```python
from build123d import *

# Parameters (mm, degrees)
BOSS_EXTRUDE1_DEPTH = 28.3
SKETCH2_W           = 52.78
SKETCH2_H           = 15.38
CUT_EXTRUDE1_DEPTH  = 10.2
CUT_EXTRUDE2_START  = 28.3
SKETCH2_2_W         = 52.78
SKETCH2_2_H         = 15.38
CUT_EXTRUDE2_DEPTH  = 10.2
CUT_EXTRUDE3_REACH  = 69.103
SKETCH3_R           = 1.65
BOSS_EXTRUDE2_START = 11.1
BOSS_EXTRUDE2_DEPTH = 3.4
CUT_EXTRUDE4_DEPTH  = 4.02
SKETCH6_R           = 1.65
BOSS_EXTRUDE3_DEPTH = 3.2
CUT_EXTRUDE5_DEPTH  = 4.22
SKETCH10_W          = 41.62
SKETCH10_H          = 8.42
CUT_EXTRUDE6_DEPTH  = 1


with BuildPart() as part:
    # Sketch1 → Boss-Extrude1 (new body)
    with BuildSketch(Plane.XY):
        with BuildLine():
            Line((0, 21.81), (3.19, 21.81))
            Line((3.19, 21.81), (3.19, 4.02))
            Line((3.19, 4.02), (53.61, 4.02))
            Line((53.61, 4.02), (53.61, 21.81))
            Line((53.61, 21.81), (56.8, 21.81))
            Line((56.8, 21.81), (56.8, 2))
            ThreePointArc((56.8, 2), (56.214213562, 0.585786438), (54.8, 0))
            Line((54.8, 0), (2, 0))
            ThreePointArc((2, 0), (0.585786438, 0.585786438), (0, 2))
            Line((0, 2), (0, 21.81))
        make_face()
    extrude(amount=BOSS_EXTRUDE1_DEPTH)

    # Sketch2 → Cut-Extrude1 (cut)
    with BuildSketch(Plane.XY):
        with Locations((28.4, 11.71)):
            Rectangle(SKETCH2_W, SKETCH2_H)
    extrude(amount=CUT_EXTRUDE1_DEPTH, mode=Mode.SUBTRACT)

    # Sketch2<2> → Cut-Extrude2 (cut)
    with BuildSketch(Plane.XY.offset(CUT_EXTRUDE2_START)):
        with Locations((28.4, 11.71)):
            Rectangle(SKETCH2_2_W, SKETCH2_2_H)
    extrude(amount=-CUT_EXTRUDE2_DEPTH, mode=Mode.SUBTRACT)

    # Cut-Extrude3: up to this face of the body (flat: up to its plane)
    cut_extrude3_end = Plane(part.part.faces().sort_by_distance((56.8, 11.905, 14.15))[0])
    # Sketch3 → Cut-Extrude3 (cut, up to the picked face)
    with BuildSketch(Plane.ZY, mode=Mode.PRIVATE) as cut_extrude3_sk1:
        with Locations((3.9, 8.91)):
            Circle(SKETCH3_R)
    cut_extrude3_tool1 = split(extrude(cut_extrude3_sk1.sketch, amount=-CUT_EXTRUDE3_REACH, mode=Mode.PRIVATE), bisect_by=cut_extrude3_end, keep=Keep.BOTH, mode=Mode.PRIVATE)
    # Sketch3 → Cut-Extrude3 (cut, up to the picked face)
    with BuildSketch(Plane.ZY, mode=Mode.PRIVATE) as cut_extrude3_sk2:
        with Locations((24.4, 8.91)):
            Circle(SKETCH3_R)
    cut_extrude3_tool2 = split(extrude(cut_extrude3_sk2.sketch, amount=-CUT_EXTRUDE3_REACH, mode=Mode.PRIVATE), bisect_by=cut_extrude3_end, keep=Keep.BOTH, mode=Mode.PRIVATE)
    add(cut_extrude3_tool1.solids().sort_by(Axis((0, 8.91, 3.9), (1, 0, 0)))[0], mode=Mode.SUBTRACT)
    add(cut_extrude3_tool2.solids().sort_by(Axis((0, 8.91, 24.4), (1, 0, 0)))[0], mode=Mode.SUBTRACT)

    # Sketch4 → Boss-Extrude2 (add)
    with BuildSketch(Plane.XY.offset(BOSS_EXTRUDE2_START)):
        with BuildLine():
            Line((8.612132034, 9.286042559), (13.378174593, 4.52))
            Line((13.378174593, 4.52), (43.421825407, 4.52))
            Line((43.421825407, 4.52), (48.187867966, 9.286042559))
            ThreePointArc((48.187867966, 9.286042559), (48.51480503, 9.351074384), (48.7, 9.073910524))
            Line((48.7, 9.073910524), (48.7, 4.02))
            Line((48.7, 4.02), (8.1, 4.02))
            Line((8.1, 4.02), (8.1, 9.073910524))
            ThreePointArc((8.1, 9.073910524), (8.28519497, 9.351074384), (8.612132034, 9.286042559))
        make_face()
    extrude(amount=BOSS_EXTRUDE2_DEPTH)

    # Sketch5 → Cut-Extrude4 (cut)
    with BuildSketch(Plane.XZ):
        with BuildLine():
            Line((5.229437252, 28.3), (39.170562748, 28.3))
            ThreePointArc((39.170562748, 28.3), (22.2, 20.3), (5.229437252, 28.3))
        make_face()
    extrude(amount=-CUT_EXTRUDE4_DEPTH, mode=Mode.SUBTRACT)

    # Sketch6 → Boss-Extrude3 (add)
    # profile 1 of 2: a face of its own
    with BuildSketch(Plane.XZ):
        with BuildLine():
            Line((9.09, 1), (23.9, 1))
            ThreePointArc((23.9, 1), (24.960660172, 1.439339828), (25.4, 2.5))
            Line((25.4, 2.5), (25.4, 7.5))
            ThreePointArc((25.4, 7.5), (24.960660172, 8.560660172), (23.9, 9))
            Line((23.9, 9), (9.09, 9))
            ThreePointArc((9.09, 9), (8.029339828, 8.560660172), (7.59, 7.5))
            Line((7.59, 7.5), (7.59, 2.5))
            ThreePointArc((7.59, 2.5), (8.029339828, 1.439339828), (9.09, 1))
        make_face()
        with Locations(Location((20.4, 5, 0), (0, 0, 270))):
            Circle(SKETCH6_R, mode=Mode.SUBTRACT)
        with Locations(Location((12.59, 5, 0), (0, 0, 270))):
            Circle(SKETCH6_R, mode=Mode.SUBTRACT)
    # profile 2 of 2: a face of its own
    with BuildSketch(Plane.XZ):
        with BuildLine():
            Line((32.9, 9), (47.71, 9))
            ThreePointArc((47.71, 9), (48.770660172, 8.560660172), (49.21, 7.5))
            Line((49.21, 7.5), (49.21, 2.5))
            ThreePointArc((49.21, 2.5), (48.770660172, 1.439339828), (47.71, 1))
            Line((47.71, 1), (32.9, 1))
            ThreePointArc((32.9, 1), (31.839339828, 1.439339828), (31.4, 2.5))
            Line((31.4, 2.5), (31.4, 7.5))
            ThreePointArc((31.4, 7.5), (31.839339828, 8.560660172), (32.9, 9))
        make_face()
        with Locations(Location((36.4, 5, 0), (0, 0, 270))):
            Circle(SKETCH6_R, mode=Mode.SUBTRACT)
        with Locations(Location((44.21, 5, 0), (0, 0, 270))):
            Circle(SKETCH6_R, mode=Mode.SUBTRACT)
    extrude(amount=BOSS_EXTRUDE3_DEPTH)

    # Sketch8 → Cut-Extrude5 (cut)
    with BuildSketch(Plane.XZ.offset(-4.02)):
        Polygon((23.3, 6.674315781), (20.4, 8.348631561), (17.5, 6.674315781), (17.5, 3.325684219), (20.4, 1.651368439), (23.3, 3.325684219), align=None)
        Polygon((39.3, 6.674315781), (36.4, 8.348631561), (33.5, 6.674315781), (33.5, 3.325684219), (36.4, 1.651368439), (39.3, 3.325684219), align=None)
        Polygon((47.11, 6.674315781), (44.21, 8.348631561), (41.31, 6.674315781), (41.31, 3.325684219), (44.21, 1.651368439), (47.11, 3.325684219), align=None)
        Polygon((15.49, 6.674315781), (12.59, 8.348631561), (9.69, 6.674315781), (9.69, 3.325684219), (12.59, 1.651368439), (15.49, 3.325684219), align=None)
    extrude(amount=CUT_EXTRUDE5_DEPTH, mode=Mode.SUBTRACT)

    # Sketch10 → Cut-Extrude6 (cut)
    with BuildSketch(Plane(origin=(0, 0, 0), x_dir=(-1, 0, 0), z_dir=(0, 0, -1))):
        with Locations((-28.4, -0.19)):
            Rectangle(SKETCH10_W, SKETCH10_H)
    extrude(amount=-CUT_EXTRUDE6_DEPTH, mode=Mode.SUBTRACT)


solid = part.part
```
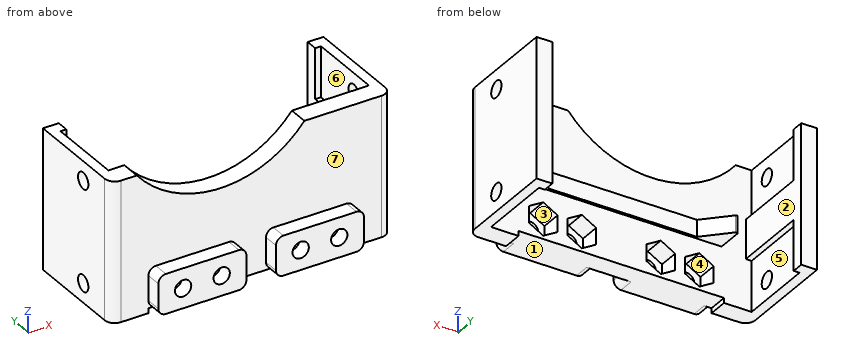
For this review, take the finished solid that the model builds, in its own axes (mm). Face numbers are marked on the shaded views. A direction names the side the tool comes from. Round coordinates to 2 decimals unless told otherwise and drop trailing zeros. Write each loop counter-clockwise with the first axis right and the second up, starting at its lowest first coordinate (ties: lowest second). Pieces come first, ordered by that corner, then holes. Notation, with made-up numbers: (89, 57) -> (141, 57) arc R23 ccw to (141, 95) -> close; hole circle Ø4 at (87.25, -30). An arc over 180 degrees is marked (long way). One line per question, with ' | ' between items. Start each with the question number.
1) Mouldability with a two-part tool opening along Y and no side actions: class the marked faces 4, 5, 6 and 7 as +Y half, -Y half, draft (parallel to the pull), parting line (faces both ways), or undercut.
2) Add section C-C (z = 24.4). Write out the cut boundary in (x, y), and give its area (3 significant figures).
3) Add section B-B (y = 12.75). Write out the cut boundary in (x, z), and give its area (3 significant figures).
4) Add section D-D (x = 26.5). Write out the cut boundary in (y, z).
5) For pin 1 Ø1.3 at (x, z) = (54.5, 5) entering from -Y; pin 2 Ø1 at (x, z) = (7.5, 18) entering from +Y; pin 3 Ø2.5 at (x, y) = (15, -2) entering from +Z, all flat-tipped, find the tip position at first contact; note any pin that passes through.
6) Add section A-A (y = -0.75). Write out the cut boundary in (x, z).
7) Wall thickness on line 1 along X through (y, z) = (-2.25, 5); line 2 along X through (y, z) = (17.75, 18); line 3 along X through (y, z) = (11.75, 4.25): over which ranges is each line inside the solid? List them lowest first.
8) Machinability: for the marked faces 1, 2 and 3, which of the approach directions +Z, -Z, +X, -X, +Y, -Y give a long, thin tool a straight path to every point of the face, cutting with its end or side? Answer none if there is none.
Reported:
1) face 4: draft | face 5: undercut | face 6: undercut | face 7: -Y half
2) outline: (0, 2) arc R2 ccw to (2, 0) -> (9.41, 0) -> (9.41, 4.02) -> (2.01, 4.02) -> (2.01, 7.26) -> (0, 7.26) -> close; (0, 10.56) -> (2.01, 10.56) -> (2.01, 19.4) -> (3.19, 19.4) -> (3.19, 21.81) -> (0, 21.81) -> close; (34.99, 0) -> (54.8, 0) arc R2 ccw to (56.8, 2) -> (56.8, 7.26) -> (54.79, 7.26) -> (54.79, 4.02) -> (34.99, 4.02) -> close; (53.61, 19.4) -> (54.79, 19.4) -> (54.79, 10.56) -> (56.8, 10.56) -> (56.8, 21.81) -> (53.61, 21.81) -> close | area: 188 mm²
3) outline: (0, 0) -> (2.01, 0) -> (2.01, 10.2) -> (3.19, 10.2) -> (3.19, 18.1) -> (2.01, 18.1) -> (2.01, 28.3) -> (0, 28.3) -> close; (53.61, 10.2) -> (54.79, 10.2) -> (54.79, 0) -> (56.8, 0) -> (56.8, 28.3) -> (54.79, 28.3) -> (54.79, 18.1) -> (53.61, 18.1) -> close | area: 132 mm²
4) outline: (0, 1) -> (4.02, 1) -> (4.02, 11.1) -> (4.52, 11.1) -> (4.52, 14.5) -> (4.02, 14.5) -> (4.02, 20.72) -> (0, 20.72) -> close
5) pin 1: stops at y = 0 | pin 2: stops at y = 4.02 | pin 3: stops at z = 9
6) outline: (7.59, 2.5) arc R1.5 ccw to (9.09, 1) -> (23.9, 1) arc R1.5 ccw to (25.4, 2.5) -> (25.4, 7.5) arc R1.5 ccw to (23.9, 9) -> (9.09, 9) arc R1.5 ccw to (7.59, 7.5) -> close; (31.4, 2.5) arc R1.5 ccw to (32.9, 1) -> (47.71, 1) arc R1.5 ccw to (49.21, 2.5) -> (49.21, 7.5) arc R1.5 ccw to (47.71, 9) -> (32.9, 9) arc R1.5 ccw to (31.4, 7.5) -> close; hole circle Ø3.3 at (12.59, 5); hole circle Ø3.3 at (20.4, 5); hole circle Ø3.3 at (36.4, 5); hole circle Ø3.3 at (44.21, 5)
7) line 1: x = 7.59 to 10.94, 14.24 to 18.75, 22.05 to 25.4, 31.4 to 34.75, 38.05 to 42.56, 45.86 to 49.21 | line 2: x = 0 to 3.19, 53.61 to 56.8 | line 3: x = 0 to 2.01, 54.79 to 56.8
8) face 1: -Z, +Y, -Y | face 2: +Z, -Z, +Y | face 3: +Y
